Part model, mm, in its own coordinate system. A direction names the side the tool comes from. Round coordinates to 2 decimals unless told otherwise and drop trailing zeros. Write each loop counter-clockwise with the first axis right and the second up, starting at its lowest first coordinate (ties: lowest second). Pieces come first, ordered by that corner, then holes. Notation, with made-up numbers: M 55,44 L 84,44 A9 cw 84,56 Z; hole C -36.5,76.25 d8. An arc over 180 degrees is marked long. Use a Markdown table: item, result. Add a question column.
1) Wall check: probe 1 along Z at (x, y) = (-2.5, 1.25); probe 2 along Y at (x, z) = (-4, -0.7); probe 3 along X at (y, z) = (-2.5, -1.15). Give the ranges that are in metal, low to high.
2) Drop flat-ended pins along their axis: P1, Ø5, axis at x = 4.5, y = -3.5, coming from the +Z side; P2, Ø1, axis at x = 1.5, z = -2, coming from the -Y side; P3, Ø1, axis at y = -5, z = 0, coming from the -X side. Give the stop position or say it passes through.
3) Slice it at B-B on z = -0.9. Write the cut outline in (x, y), plus the area to 3 significant figures.
4) Which spindle directions (+Z, -Z, +X, -X, +Y, -Y) get a long thin tool onto all of the face, cutting with end or side? Do faces 1 (the face through (0, -3, 0)), 2 (the face through (-1.38, -6.2, -1.51)), 3 (the face through (0, 3, 0)). Say none if no direction does.
5) Two-plate mould, pull along Y, no slides. Class faces 4 (the face through (-5.843, -0.257, -0.007)), 5 (the face through (0, 0, -2.54)): released by +Y, released by -Y, zero draft, split by the parting line, or undercut.
6) Slice it at A-A on x = 0. Write the cut outline in (y, z), plus the area to 3 significant figures.
```python
from build123d import *

# Parameters (mm, degrees)
F3_DEPTH = 6.35
F0_R     = 6.35
F4_DEPTH = 2.54
F5_R     = 12.7
F5_R_2   = 6.35
F6_DEPTH = 6.35


with BuildPart() as f3:
    # F2 (on Right) → F3 (new body, symmetric)
    with BuildSketch(Plane.YZ):
        Polygon((0, -0.508), (0.508, 0), (0, 0.508), (-0.508, 0), align=None)
    extrude(amount=F3_DEPTH, both=True)

    # F0 (on Top) → F4 (join)
    with BuildSketch(Plane.XY):
        Circle(F0_R)
    extrude(amount=-F4_DEPTH)

    # F5 (on face) → F6 (cut, symmetric)
    with BuildSketch(Plane.XY):
        Circle(F5_R)
        Circle(F5_R_2, mode=Mode.SUBTRACT)
    extrude(amount=F6_DEPTH, both=True, mode=Mode.SUBTRACT)

    # F7 (on Front) → F8 (revolve, cut)
    with BuildSketch(Plane.XZ):
        Polygon((6.35, 0.508), (5.334, 0.508), (6.35, -0.508), align=None)
    revolve(axis=Axis((0, 0, -0.254), (0, 0, -1)), mode=Mode.SUBTRACT)


solid = f3.part
```
Entries:
| question | item | result |
|---|---|---|
| 1 | probe 1 | z = -2.54 to 0 |
| 1 | probe 2 | y = -4.93 to 4.93 |
| 1 | probe 3 | x = -5.84 to 5.84 |
| 2 | P1 | stops at z = 0 |
| 2 | P2 | stops at y = -6.27 |
| 2 | P3 | stops at x = -4.11 |
| 3 | outline | C 0,0 d12.7 |
| 3 | area | 127 mm^2 |
| 4 | face 1 | +Z, +X, -X, -Y |
| 4 | face 2 | +Z, -Z |
| 4 | face 3 | +Z, +X, -X, +Y |
| 5 | face 4 | split by the parting line |
| 5 | face 5 | zero draft |
| 6 | outline | M -6.35,-2.54 L 6.35,-2.54 L 6.35,-0.51 L 5.84,0 L 0.51,0 L 0,0.51 L -0.51,0 L -5.84,0 L -6.35,-0.51 Z |
| 6 | area | 32.3 mm^2 |
